Could you check a few things on this model? Use its own coordinates, in mm. Give positions to 0.01 mm unless a question says otherwise; leave off trailing zeros. Order: outer loops, then holes, each group sorted by start corner. A loop starts at its lowest first (then second) coordinate and runs counter-clockwise, first axis right, second up.
from build123d import *

# Parameters (mm, degrees)
SKETCH_1_R      = 25
SKETCH_1_R_2    = 1.1
SKETCH_1_R_3    = 1.65
EXTRUDE_1_DEPTH = 3


with BuildPart() as part:
    # 草图1 → 凸台-拉伸1 (new body)
    with BuildSketch(Plane(origin=(0, 0, 0), x_dir=(1, 0, 0), z_dir=(0, 1, 0))):
        with Locations(Location((0, 0, 0), (0, 0, 270))):
            Circle(SKETCH_1_R)
        with Locations(Location((0, 12, 0), (0, 0, 270))):
            Circle(SKETCH_1_R_2, mode=Mode.SUBTRACT)
        with Locations(Location((-9.25, 16.02146997, 0), (0, 0, 270))):
            Circle(SKETCH_1_R_3, mode=Mode.SUBTRACT)
        with Locations(Location((9.25, 16.02146997, 0), (0, 0, 270))):
            Circle(SKETCH_1_R_3, mode=Mode.SUBTRACT)
        with Locations(Location((10.392304845, 6, 0), (0, 0, 270))):
            Circle(SKETCH_1_R_2, mode=Mode.SUBTRACT)
        with Locations(Location((18.5, 0, 0), (0, 0, 270))):
            Circle(SKETCH_1_R_3, mode=Mode.SUBTRACT)
        with Locations(Location((10.392304845, -6, 0), (0, 0, 270))):
            Circle(SKETCH_1_R_2, mode=Mode.SUBTRACT)
        with Locations(Location((9.25, -16.02146997, 0), (0, 0, 270))):
            Circle(SKETCH_1_R_3, mode=Mode.SUBTRACT)
        with Locations(Location((0, -12, 0), (0, 0, 270))):
            Circle(SKETCH_1_R_2, mode=Mode.SUBTRACT)
        with Locations(Location((-9.25, -16.02146997, 0), (0, 0, 270))):
            Circle(SKETCH_1_R_3, mode=Mode.SUBTRACT)
        with Locations(Location((-10.392304845, -6, 0), (0, 0, 270))):
            Circle(SKETCH_1_R_2, mode=Mode.SUBTRACT)
        with Locations(Location((-18.5, 0, 0), (0, 0, 270))):
            Circle(SKETCH_1_R_3, mode=Mode.SUBTRACT)
        with Locations(Location((-10.392304845, 6, 0), (0, 0, 270))):
            Circle(SKETCH_1_R_2, mode=Mode.SUBTRACT)
        with BuildLine():
            Line((-4.958957038, -1.191110864), (-0.311901361, -5.090453569))
            ThreePointArc((-0.311901361, -5.090453569), (3.278216809, 3.90682666), (-4.958957038, -1.191110864))
        make_face(mode=Mode.SUBTRACT)
    extrude(amount=EXTRUDE_1_DEPTH)


solid = part.part
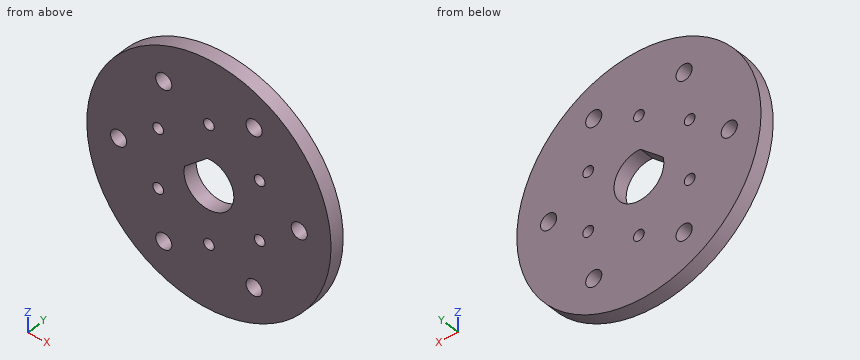
Item 1: Imagine slicing it at C-C on z = 17. List the corners of the cut face in (x, y) for me, then the cut area to 3 significant figures.
Findings:
outline: (-18.33, 0) - (-10.58, 0) - (-10.58, 3) - (-18.33, 3) - close; (-7.92, 0) - (7.92, 0) - (7.92, 3) - (-7.92, 3) - close; (10.58, 0) - (18.33, 0) - (18.33, 3) - (10.58, 3) - close
area: 94.0 mm2
Item 2: Please list where these lines run through material, in increasing order: line 1 along X through (y, z) = (2.15, 0); line 2 along X through (y, z) = (1.1, 1.5); line 3 along X through (y, z) = (1.05, -6).
Findings:
line 1: x = -25 to -20.15, -16.85 to -5.1, 5.1 to 16.85, 20.15 to 25
line 2: x = -24.95 to -19.19, -17.81 to -4.59, 4.87 to 17.81, 19.19 to 24.95
line 3: x = -24.27 to -11.49, -9.29 to 9.29, 11.49 to 24.27
Item 3: For pin 1 (1.3 mm diameter, centred on x = 0, z = -12, fed in from +Y), with a flat end and sliding along its axis, tell me the tip position at first contact or that it passes through.
Findings:
pin 1: passes through
Item 4: Imagine slicing it at B-B on x = -18.5. List the corners of the cut face in (y, z) for me, then the cut area to 3 significant figures.
Findings:
outline: (0, -16.82) - (3, -16.82) - (3, -1.65) - (0, -1.65) - close; (0, 1.65) - (3, 1.65) - (3, 16.82) - (0, 16.82) - close
area: 91.0 mm2
Item 5: Imagine slicing it at D-D on y = 0.65. Give the number of separate pieces and of enclosed holes in the cut face, then the cut area to 3 significant figures.
Findings:
separate pieces: 1
enclosed holes: 13
area: 1,810 mm2
Item 6: Imagine slicing it at A-A on z = 0. List the corners of the cut face in (x, y) for me.
Findings:
outline: (-25, 0) - (-20.15, 0) - (-20.15, 3) - (-25, 3) - close; (-16.85, 0) - (-5.1, 0) - (-5.1, 3) - (-16.85, 3) - close; (5.1, 0) - (16.85, 0) - (16.85, 3) - (5.1, 3) - close; (20.15, 0) - (25, 0) - (25, 3) - (20.15, 3) - close
